```python
from build123d import *

# Parameters (mm, degrees)
SKETCH1_W           = 7
SKETCH1_H           = 40
BOSS_EXTRUDE1_DEPTH = 3.175
SKETCH2_W           = 7
SKETCH2_H           = 40
SKETCH2_R           = 2
BOSS_EXTRUDE2_DEPTH = 3.175


with BuildPart() as part:
    # Sketch1 → Boss-Extrude1 (new body)
    with BuildSketch(Plane(origin=(0, 0, 0), x_dir=(1, 0, 0), z_dir=(0, 1, 0))):
        Rectangle(SKETCH1_W, SKETCH1_H)
    extrude(amount=BOSS_EXTRUDE1_DEPTH)

    # Sketch2 → Boss-Extrude2 (add)
    with BuildSketch(Plane(origin=(0, 3.175, 0), x_dir=(1, 0, 0), z_dir=(0, 1, 0))):
        Rectangle(SKETCH2_W, SKETCH2_H)
        with Locations(Location((0, 16, 0), (0, 0, 270))):
            Circle(SKETCH2_R, mode=Mode.SUBTRACT)
        with Locations(Location((0, -16, 0), (0, 0, 270))):
            Circle(SKETCH2_R, mode=Mode.SUBTRACT)
    extrude(amount=BOSS_EXTRUDE2_DEPTH)


solid = part.part
```
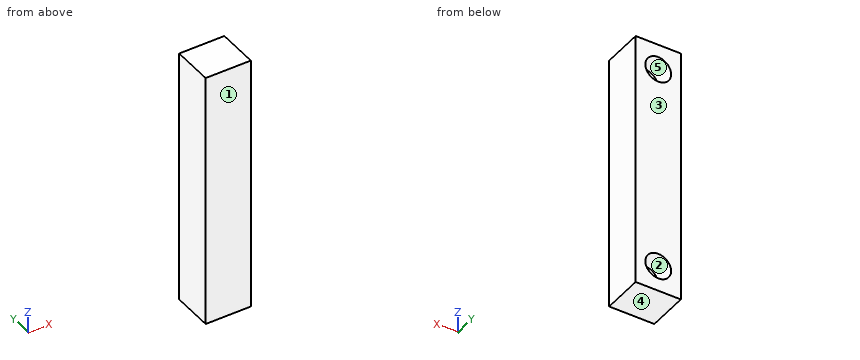
Geometry: final body of the model. Coordinates: model frame, mm. Face numbers are marked on the shaded views. A direction names the side the tool comes from. Round coordinates to 2 decimals unless told otherwise and drop trailing zeros. Loops run counter-clockwise (first coordinate to the right, second up) from the corner with the lowest first, then second, coordinate; pieces in that order, holes last.
Item 1: Section A-A, the plane z = 16. Output: boundary loops of the cut face in (x, y) (3 decimals), plus the area to 4 significant figures.
Checked values:
outline: (-3.5, 0) - (3.5, 0) - (3.5, 6.35) - (2, 6.35) - (2, 3.175) - (-2, 3.175) - (-2, 6.35) - (-3.5, 6.35) - close
area: 31.75 mm2
Item 2: Mould query, pull axis Z, two halves, no side actions, for the marked faces 3, 4 and 5. Classes: released by +Z, released by -Z, zero draft, split by the parting line, or undercut.
Checked values:
face 3: zero draft
face 4: released by -Z
face 5: undercut
Item 3: Section B-B, the plane y = 4.5. Output: boundary loops of the cut face in (x, z).
Checked values:
outline: (-3.5, -20) - (3.5, -20) - (3.5, 20) - (-3.5, 20) - close; hole circle Ø4 at (0, -16); hole circle Ø4 at (0, 16)
Item 4: Reachability of the marked faces 1 and 2 from +Z, -Z, +X, -X, +Y, -Y: full face, straight path, thin tool, end or side. Return the list, or none.
Checked values:
face 1: +Z, -Z, +X, -X, -Y
face 2: +Y
Item 5: Section C-C, the plane x = 0. Output: boundary loops of the cut face in (y, z) (3 decimals), plus the area to 3 significant figures.
Checked values:
outline: (0, -20) - (6.35, -20) - (6.35, -18) - (3.175, -18) - (3.175, -14) - (6.35, -14) - (6.35, 14) - (3.175, 14) - (3.175, 18) - (6.35, 18) - (6.35, 20) - (0, 20) - close
area: 229 mm2
Item 6: Line query: L1, parallel to X at y = 4.25, z = -16; L2, parallel to Z at x = 1.25, y = 4; L3, parallel to Z at x = -0.25, y = 4.5. Output: solid intervals per line, ascending.
Checked values:
L1: x = -3.5 to -2, 2 to 3.5
L2: z = -20 to -17.56, -14.44 to 14.44, 17.56 to 20
L3: z = -20 to -17.98, -14.02 to 14.02, 17.98 to 20
